Verification items for the finished model (mm, model axes). Face numbers are marked on the shaded views. A direction names the side the tool comes from. Coordinates: 2 decimals unless noted, no trailing zeros. Loops run counter-clockwise (first coordinate to the right, second up) from the corner with the lowest first, then second, coordinate; pieces in that order, holes last. Notation, with made-up numbers: (-20, 85.25) - (30, 85.25) arc R20 ccw to (30, 99.25) - close; hole circle Ø9 at (43.5, -39). An arc over 180 degrees is marked (long way). Answer as CSV lines item,"result". Start each with the question number.
1. Cross-section at B-B (y = 39). Enter the section's corners in (x, z).
2. Cross-section at C-C (z = 23.25). Enter the section's corners in (x, y).
3. Set-up check for the marked faces 1, 2 and 3: record each of +Z, -Z, +X, -X, +Y, -Y from which the full face is reachable in a straight line by a thin tool's end or side.
4. Gauge pin test, flat ends, axial feed: P1, Ø2, axis at x = 12, y = 11.5, coming from the +Z side; P2, Ø1.2, axis at x = 10.07, z = 12.5, coming from the +Y side; P3, Ø12, axis at x = -0.5, z = 24, coming from the +Y side. Record the tip position at first contact, or that the pin passes through.
5. Cross-section at A-A (x = 21). Enter the section's corners in (y, z).
6. Material ranges on line 1 (X direction, y = 25.5, z = 32.5); line 2 (Y direction, x = 18.5, z = 14.5); line 3 (Z direction, x = 10.5, y = -20), recorded low to high. Write a range as [from, to].
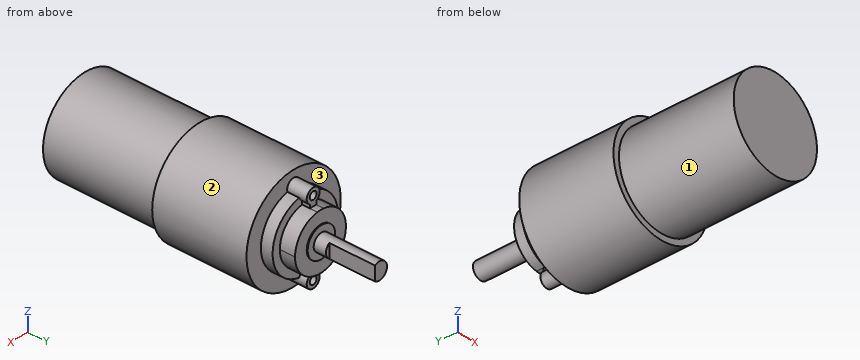
```python
from build123d import *

# Parameters (mm, degrees)
FRONT_CYLINDER_SKETCH_R    = 13.7
FRONT_CYLINDER_DEPTH       = 24.81270946
MOUNTING_POINT_SKETCH_R    = 1
MOUNTING_POINTS_DEPTH      = 5.15
GEAR_MOUNT_BOTTOM_SKETCH_R = 9.5
GEAR_MOUNT_BOTTOM_DEPTH    = 3.074685726
GEAR_MOUNT_TOP_DEPTH       = 4
MOUNTING_HOLES_REACH       = 9.075
MOUNTING_HOLES_SKETCH_R    = 1
GEAR_DISK_SKETCH_R         = 4
GEAR_DISK_DEPTH            = 0.25
GEAR_SKETCH_R              = 2.25
GEAR_DEPTH                 = 15.225
GEAR_NOTCH_DEPTH           = 12
BACK_CYLINDER_SKETCH_R     = 12.1
BOSS_EXTRUDE7_DEPTH        = 30.2


with BuildPart() as part:
    # Front cylinder sketch → Front Cylinder (new body)
    with BuildSketch(Plane(origin=(0, 0, 0), x_dir=(1, 0, 0), z_dir=(0, 1, 0))):
        with Locations((10.070944868, -22.415974061)):
            Circle(FRONT_CYLINDER_SKETCH_R)
    extrude(amount=FRONT_CYLINDER_DEPTH)

    # Mounting Point Sketch → Mounting Points (add)
    with BuildSketch(Plane(origin=(0, 24.81270946, 0), x_dir=(1, 0, 0), z_dir=(0, 1, 0))):
        with BuildLine():
            Line((10.970944868, -15.079824378), (10.970944868, -14.148518185))
            ThreePointArc((10.970944868, -14.148518185), (10.070944868, -10.614245578), (9.170944868, -14.148518185))
            Line((9.170944868, -14.148518185), (9.170944868, -15.079824378))
            ThreePointArc((9.170944868, -15.079824378), (10.070944868, -15.024824478), (10.970944868, -15.079824378))
        make_face()
        with Locations((10.070944868, -12.495974061)):
            Circle(MOUNTING_POINT_SKETCH_R, mode=Mode.SUBTRACT)
        with BuildLine():
            Line((9.170944868, -29.752123743), (9.170944868, -30.683429936))
            ThreePointArc((9.170944868, -30.683429936), (10.070944868, -34.217702543), (10.970944868, -30.683429936))
            Line((10.970944868, -30.683429936), (10.970944868, -29.752123743))
            ThreePointArc((10.970944868, -29.752123743), (10.070944868, -29.807123644), (9.170944868, -29.752123743))
        make_face()
        with Locations((10.070944868, -32.335974061)):
            Circle(MOUNTING_POINT_SKETCH_R, mode=Mode.SUBTRACT)
    extrude(amount=MOUNTING_POINTS_DEPTH)

    # Gear Mount Bottom Sketch → Gear Mount Bottom (add)
    with BuildSketch(Plane(origin=(0, 24.81270946, 0), x_dir=(1, 0, 0), z_dir=(0, 1, 0))):
        with Locations((10.070944868, -22.415974061)):
            Circle(GEAR_MOUNT_BOTTOM_SKETCH_R)
    extrude(amount=GEAR_MOUNT_BOTTOM_DEPTH)

    # Gear Mount Top Sketch → Gear Mount Top (add)
    with BuildSketch(Plane(origin=(0, 27.887395186, 0), x_dir=(1, 0, 0), z_dir=(0, 1, 0))):
        with BuildLine():
            ThreePointArc((17.462094451, -22.415974061), (15.606336759, -17.518165493), (10.970944868, -15.079824378))
            ThreePointArc((10.970944868, -15.079824378), (10.070944868, -15.024824478), (9.170944868, -15.079824378))
            ThreePointArc((9.170944868, -15.079824378), (2.679795285, -22.415974061), (9.170944868, -29.752123743))
            ThreePointArc((9.170944868, -29.752123743), (10.070944868, -29.807123644), (10.970944868, -29.752123743))
            ThreePointArc((10.970944868, -29.752123743), (15.606336759, -27.313782629), (17.462094451, -22.415974061))
        make_face()
    extrude(amount=GEAR_MOUNT_TOP_DEPTH)

    # Mounting Holes Sketch → Mounting Holes (cut, up to next)
    with BuildSketch(Plane(origin=(0, 24.81270946, 0), x_dir=(1, 0, 0), z_dir=(0, 1, 0)), mode=Mode.PRIVATE) as mounting_holes_sk1:
        with Locations((10.070944868, -12.495974061)):
            Circle(MOUNTING_HOLES_SKETCH_R)
    mounting_holes_tool1 = extrude(mounting_holes_sk1.sketch, amount=MOUNTING_HOLES_REACH, mode=Mode.PRIVATE) & part.part
    add(mounting_holes_tool1.solids().sort_by_distance((10.070945, 24.812709, 12.495974))[0], mode=Mode.SUBTRACT)
    # Mounting Holes Sketch → Mounting Holes (cut, up to next)
    with BuildSketch(Plane(origin=(0, 24.81270946, 0), x_dir=(1, 0, 0), z_dir=(0, 1, 0)), mode=Mode.PRIVATE) as mounting_holes_sk2:
        with Locations((10.070944868, -32.335974061)):
            Circle(MOUNTING_HOLES_SKETCH_R)
    mounting_holes_tool2 = extrude(mounting_holes_sk2.sketch, amount=MOUNTING_HOLES_REACH, mode=Mode.PRIVATE) & part.part
    add(mounting_holes_tool2.solids().sort_by_distance((10.070945, 24.812709, 32.335974))[0], mode=Mode.SUBTRACT)

    # Gear Disk Sketch → Gear disk (add)
    with BuildSketch(Plane(origin=(0, 31.887395186, 0), x_dir=(1, 0, 0), z_dir=(0, 1, 0))):
        with Locations((10.070944868, -22.415974061)):
            Circle(GEAR_DISK_SKETCH_R)
    extrude(amount=GEAR_DISK_DEPTH)

    # Gear Sketch → Gear (add)
    with BuildSketch(Plane(origin=(0, 32.137395186, 0), x_dir=(1, 0, 0), z_dir=(0, 1, 0))):
        with Locations((10.070944868, -22.415974061)):
            Circle(GEAR_SKETCH_R)
    extrude(amount=GEAR_DEPTH)

    # Gear Notch Sketch → Gear Notch (cut)
    with BuildSketch(Plane(origin=(0, 47.362395186, 0), x_dir=(1, 0, 0), z_dir=(0, 1, 0))):
        with BuildLine():
            ThreePointArc((12.320944868, -22.415974061), (12.055258351, -21.355313889), (11.320944868, -20.545145367))
            Line((11.320944868, -20.545145367), (11.320944868, -24.286802754))
            ThreePointArc((11.320944868, -24.286802754), (12.055258351, -23.476634232), (12.320944868, -22.415974061))
        make_face()
    extrude(amount=-GEAR_NOTCH_DEPTH, mode=Mode.SUBTRACT)

    # Back Cylinder Sketch → Boss-Extrude7 (add)
    with BuildSketch(Plane.XZ):
        with Locations((10.070944868, 22.415974061)):
            Circle(BACK_CYLINDER_SKETCH_R)
    extrude(amount=BOSS_EXTRUDE7_DEPTH)


solid = part.part
```
Values follow:
1,outline,"(11.32, 20.55) - (11.32, 24.29) arc R2.25 ccw (long way) to start"
2,outline,"(-3.6, 0) - (-2, 0) - (-2, -30.2) - (22.14, -30.2) - (22.14, 0) - (23.75, 0) - (23.75, 24.81) - (19.53, 24.81) - (19.53, 27.89) - (17.41, 27.89) - (17.41, 31.89) - (13.98, 31.89) - (13.98, 32.14) - (12.16, 32.14) - (12.16, 35.36) - (11.32, 35.36) - (11.32, 47.36) - (7.98, 47.36) - (7.98, 32.14) - (6.16, 32.14) - (6.16, 31.89) - (2.73, 31.89) - (2.73, 27.89) - (0.61, 27.89) - (0.61, 24.81) - (-3.6, 24.81) - close"
3,face 1,"-Y"
3,face 2,"+Y, -Y"
3,face 3,"+Y"
4,P1,"stops at z = 36.08"
4,P2,"stops at y = 24.81"
4,P3,"stops at y = 31.89"
5,outline,"(-30.2, 17.22) - (0, 17.22) - (0, 14.15) - (24.81, 14.15) - (24.81, 30.68) - (0, 30.68) - (0, 27.61) - (-30.2, 27.61) - close"
6,line 1,"x = [8.2, 9.08], [11.06, 11.95]"
6,line 2,"y = [-30.2, 24.81]"
6,line 3,"z = [10.32, 34.51]"
